```python
from build123d import *

# Parameters (mm, degrees)
CROQUIS1_W              = 27
CROQUIS1_H              = 12
SALIENTE_EXTRUIR1_DEPTH = 20
CROQUIS2_W              = 23
CROQUIS2_H              = 8
CORTAR_EXTRUIR1_DEPTH   = 20
REDONDEO1_R             = 3
REDONDEO2_R             = 1


with BuildPart() as part:
    # Croquis1 → Saliente-Extruir1 (new body)
    with BuildSketch(Plane.XY):
        Rectangle(CROQUIS1_W, CROQUIS1_H)
    extrude(amount=SALIENTE_EXTRUIR1_DEPTH)

    # Croquis2 → Cortar-Extruir1 (cut)
    with BuildSketch(Plane.XY.offset(20)):
        Rectangle(CROQUIS2_W, CROQUIS2_H)
    extrude(amount=-CORTAR_EXTRUIR1_DEPTH, mode=Mode.SUBTRACT)

    # Redondeo1
    redondeo1_edges = [part.edges().sort_by_distance(p)[0] for p in [
        (-13.5, 6, 10),
        (-13.5, -6, 10),
        (13.5, -6, 10),
        (13.5, 6, 10),
    ]]
    fillet(redondeo1_edges, radius=REDONDEO1_R)

    # Redondeo2
    redondeo2_edges = [part.edges().sort_by_distance(p)[0] for p in [
        (11.5, 4, 10),
        (11.5, -4, 10),
        (-11.5, -4, 10),
        (-11.5, 4, 10),
    ]]
    fillet(redondeo2_edges, radius=REDONDEO2_R)


solid = part.part
```
The listing builds one solid part. Answer for the finished solid, in the listing's coordinates (mm). A direction names the side the tool comes from. Give positions to 0.01 mm unless a question says otherwise; leave off trailing zeros. Write each loop counter-clockwise with the first axis right and the second up, starting at its lowest first coordinate (ties: lowest second). Pieces come first, ordered by that corner, then holes. Notation, with made-up numbers: (-13, 88.25) - (-8, 88.25) arc R10 ccw to (-8, 98.25) - close; hole circle Ø9 at (11.25, 27.25). An arc over 180 degrees is marked (long way). Use one line per item in the form item = value. Start each with the question number.
1) Find section C-C on z = 8.25. Determine the outline of the cut face in (x, y), plus the area to 3 significant figures.
2) A tool of negligible diameter and unlimited length cuts with its end or side. For faces 5 (the face through (11.215, 3.699, 9.86)), 6 (the face through (-12.64, 5.1, 10.14)), from which of +Z, -Z, +X, -X, +Y, -Y can it reach the whole face along a straight path? Write none if from no direction.
3) Find section D-D on y = 5. Determine the outline of the cut face in (x, z), plus the area to 3 significant figures.
4) Find section A-A on y = -2.5. Determine the outline of the cut face in (x, z).
5) Find section B-B on x = -1.25. Determine the outline of the cut face in (y, z).
6) The mould has two halves that part along Y. Classify faces 1 (the face through (0, 6, 10)), 2 (the face through (0, 5, 20)), 3 (the face through (-11.199, 3.715, 9.86)), 4 (the face through (0, -6, 10)): pulls with the +Y half, pulls with the -Y half, needs draft (parallel to the pull), parting line crosses it, or undercut.
7) Consider line 1 along Y through (x, z) = (-9.5, 14.5); line 2 along X through (y, z) = (0.25, 1); line 3 along X through (y, z) = (3.5, 12). Determine where each line is inside the solid, lowest interval first. Write a range as from..to.
Geometry results:
q1.outline = (-13.5, -3) arc R3 ccw to (-10.5, -6) - (10.5, -6) arc R3 ccw to (13.5, -3) - (13.5, 3) arc R3 ccw to (10.5, 6) - (-10.5, 6) arc R3 ccw to (-13.5, 3) - close; hole (-11.5, -3) arc R1 ccw to (-10.5, -4) - (10.5, -4) arc R1 ccw to (11.5, -3) - (11.5, 3) arc R1 ccw to (10.5, 4) - (-10.5, 4) arc R1 ccw to (-11.5, 3) - close
q1.area = 133 mm2
q2.face_5 = +Z, -Z
q2.face_6 = +Z, -Z, -X, +Y
q3.outline = (-12.74, 0) - (12.74, 0) - (12.74, 20) - (-12.74, 20) - close
q3.area = 509 mm2
q4.outline = (-13.5, 0) - (-11.5, 0) - (-11.5, 20) - (-13.5, 20) - close; (11.5, 0) - (13.5, 0) - (13.5, 20) - (11.5, 20) - close
q5.outline = (-6, 0) - (-4, 0) - (-4, 20) - (-6, 20) - close; (4, 0) - (6, 0) - (6, 20) - (4, 20) - close
q6.face_1 = pulls with the +Y half
q6.face_2 = needs draft
q6.face_3 = undercut
q6.face_4 = pulls with the -Y half
q7.line_1 = -6..-4, 4..6
q7.line_2 = -13.5..-11.5, 11.5..13.5
q7.line_3 = -13.46..-11.37, 11.37..13.46
